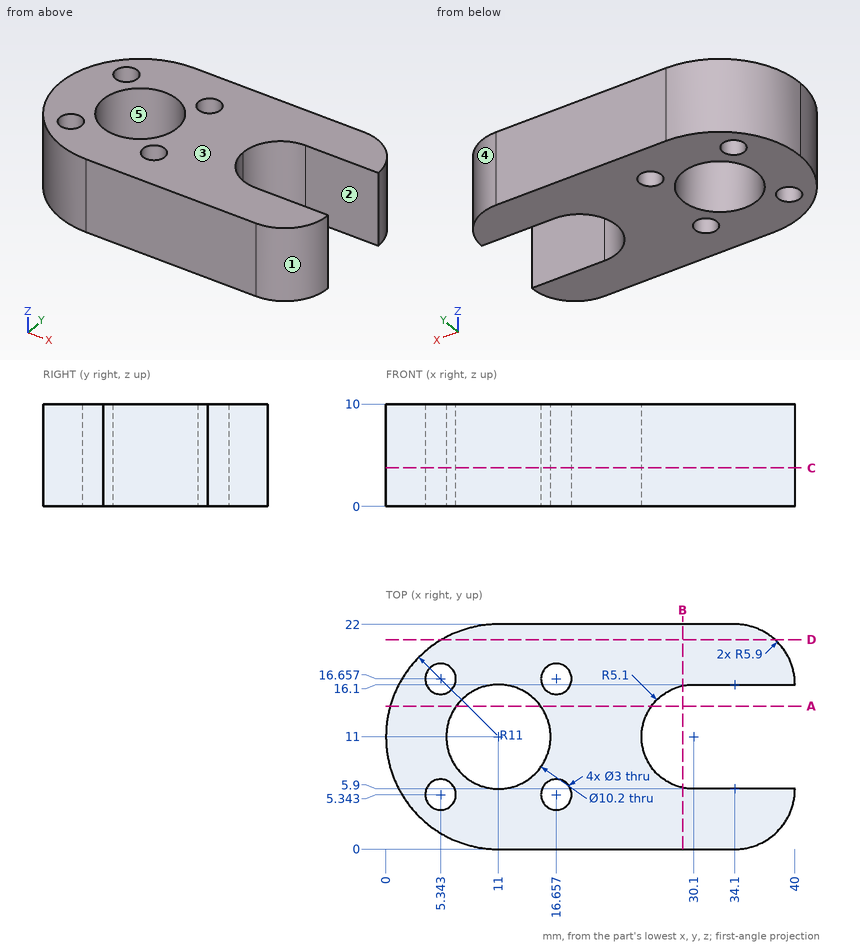
Part print with two shaded views. Sizes in mm from the minimum x, y, z corner. A direction names the side the tool comes from. Round coordinates to 2 decimals unless told otherwise and drop trailing zeros. Order: outer loops, then holes, each group sorted by start corner. A loop starts at its lowest first (then second) coordinate and runs counter-clockwise, first axis right, second up. Notation, with made-up numbers: M 29,86.5 L 50,86.5 A33 cw 50,121.5 Z; hole C -11.5,17.25 d7. An arc over 180 degrees is marked long. Use CSV: the item, a comma, the result in double quotes. Start each with the question number.
(1) Tool access for the marked faces 1 and 2: list every direction of +Z, -Z, +X, -X, +Y, -Y with a clear straight run to the whole face (end or side of a thin tool).
(2) Cut at A-A on y = 14. List the corners of the cut face in (x, z).
(3) Cut at B-B on x = 29. List the corners of the cut face in (y, z), then the cut area to 3 significant figures.
(4) Mould opens along X. For the marked faces 3, 4 and 5 say: +X half, -X half, draft (parallel to the pull), parting line (faces both ways), or undercut.
(5) Cut at D-D on y = 20.5. List the corners of the cut face in (x, z) (1 decimal), then the cut area to 3 significant figures.
(6) Flat gauge pins, fed straight in: P1, Ø1.5, axis at x = 5, z = 6.5, coming from the +Y side; P2, Ø8, axis at x = 11, y = 11, coming from the -Z side. Where does each tip first touch, or does it go through?
(7) Cut at C-C on z = 3.75. List the corners of the cut face in (x, y), then the cut area to 3 significant figures.
(8) Drill centre lines: probe 1 along Y at (x, z) = (30.5, 9.75); probe 2 along Y at (x, z) = (4, 0.5) (1 decimal); probe 3 along Y at (x, z) = (17, 2.75). Where is each one in solid material? Low to high.
Findings:
1,face 1,"+Z, -Z, +X, -Y"
1,face 2,"+Z, -Z, +X"
2,outline,"M 0.42,0 L 6.88,0 L 6.88,10 L 0.42,10 Z; M 15.12,0 L 25.98,0 L 25.98,10 L 15.12,10 Z"
3,outline,"M 0,0 L 6.02,0 L 6.02,10 L 0,10 Z; M 15.98,0 L 22,0 L 22,10 L 15.98,10 Z"
3,area,"120 mm^2"
4,face 3,"draft"
4,face 4,"+X half"
4,face 5,"undercut"
5,outline,"M 5.5,0 L 38,0 L 38,10 L 5.5,10 Z"
5,area,"326 mm^2"
6,P1,"stops at y = 20.67"
6,P2,"passes through"
7,outline,"M 0,11 A11 ccw 11,0 L 34.1,0 A5.9 ccw 40,5.9 L 30.1,5.9 A5.1 cw 25,11 A5.1 cw 30.1,16.1 L 40,16.1 A5.9 ccw 34.1,22 L 11,22 A11 ccw Z; hole C 5.34,5.34 d3; hole C 5.34,16.66 d3; hole C 11,11 d10.2; hole C 16.66,5.34 d3; hole C 16.66,16.66 d3"
7,area,"561 mm^2"
8,probe 1,"y = 0 to 5.9, 16.1 to 22"
8,probe 2,"y = 2.5 to 4.7, 6 to 16, 17.3 to 19.5"
8,probe 3,"y = 0 to 3.88, 6.8 to 15.2, 18.12 to 22"
